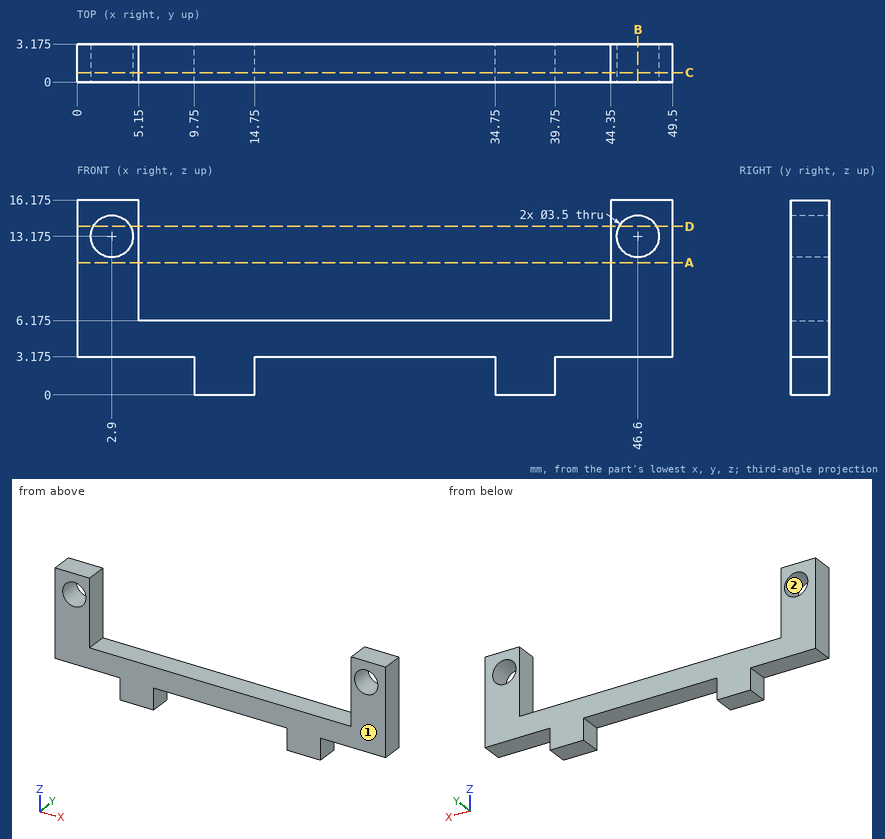
Print and shaded views of the part. All mm, measured from the part's lowest x, y and z. Give positions to 0.01 mm unless a question says otherwise; leave off trailing zeros. Loops run counter-clockwise (first coordinate to the right, second up) from the corner with the lowest first, then second, coordinate; pieces in that order, holes last.
1) Saw through at B-B (x = 46.6). Write the cut outline in (y, z) (3 decimals).
2) Wall check: line 1 (X direction, y = 1.65, z = 13); line 2 (X direction, y = 0.6, z = 9.75); line 3 (X direction, y = 0.6, z = 12). Give the ranges that are in metal, low to high.
3) Pull direction X, two halves, no side cores. Call the marked faces 1 and 2: +X half, -X half, draft (parallel to the pull), parting line (faces both ways), or undercut.
4) Saw through at D-D (z = 14). Write the cut outline in (x, y) (3 decimals).
5) Flat gauge pins, fed straight in: pin 1 Ø1.6 at (y, z) = (2, 1) entering from +X; pin 2 Ø1.6 at (y, z) = (2.5, 1) entering from -X; pin 3 Ø2 at (x, z) = (8.5, 9) entering from +Y; pin 4 Ø1 at (x, y) = (7, 1.5) entering from -Z (3 decimals). Where does each tip first touch, or does it go through?
6) Saw through at C-C (y = 0.8). Write the cut outline in (x, z) (3 decimals).
7) Saw through at A-A (z = 11). Write the cut outline in (x, y) (3 decimals).
Answer block:
1. outline: (0, 3.175) - (3.175, 3.175) - (3.175, 11.425) - (0, 11.425) - close; (0, 14.925) - (3.175, 14.925) - (3.175, 16.175) - (0, 16.175) - close
2. line 1: x = 0 to 1.16, 4.64 to 5.15, 44.35 to 44.86, 48.34 to 49.5
2. line 2: x = 0 to 5.15, 44.35 to 49.5
2. line 3: x = 0 to 1.6, 4.2 to 5.15, 44.35 to 45.3, 47.9 to 49.5
3. face 1: draft
3. face 2: undercut
4. outline: (0, 0) - (1.357, 0) - (1.357, 3.175) - (0, 3.175) - close; (4.443, 0) - (5.15, 0) - (5.15, 3.175) - (4.443, 3.175) - close; (44.35, 0) - (45.057, 0) - (45.057, 3.175) - (44.35, 3.175) - close; (48.143, 0) - (49.5, 0) - (49.5, 3.175) - (48.143, 3.175) - close
5. pin 1: stops at x = 39.75
5. pin 2: stops at x = 9.75
5. pin 3: passes through
5. pin 4: stops at z = 3.175
6. outline: (0, 3.175) - (9.75, 3.175) - (9.75, 0) - (14.75, 0) - (14.75, 3.175) - (34.75, 3.175) - (34.75, 0) - (39.75, 0) - (39.75, 3.175) - (49.5, 3.175) - (49.5, 16.175) - (44.35, 16.175) - (44.35, 6.175) - (5.15, 6.175) - (5.15, 16.175) - (0, 16.175) - close; hole circle Ø3.5 at (2.9, 13.175); hole circle Ø3.5 at (46.6, 13.175)
7. outline: (0, 0) - (5.15, 0) - (5.15, 3.175) - (0, 3.175) - close; (44.35, 0) - (49.5, 0) - (49.5, 3.175) - (44.35, 3.175) - close
